Geometry: final body of the model. Coordinates: model frame, mm. A direction names the side the tool comes from. Coordinates: 2 decimals unless noted, no trailing zeros. Loops run counter-clockwise (first coordinate to the right, second up) from the corner with the lowest first, then second, coordinate; pieces in that order, holes last. Notation, with made-up numbers: (86.5, 5) - (107.5, 5) arc R14 cw to (107.5, 28) - close; hole circle Ø6 at (-12, 47). An arc over 180 degrees is marked (long way). Answer in a Markdown table with one row per item.
from build123d import *

# Parameters (mm, degrees)
ESQUISSE1_W             = 600
ESQUISSE1_H             = 480
BOSS_EXTRU_1_DEPTH      = 18
ESQUISSE2_W             = 100
ESQUISSE2_H             = 79
ENL_V_MAT_EXTRU_1_DEPTH = 17
ENL_V_MAT_EXTRU_3_DEPTH = 10
CONG_1_R                = 2


with BuildPart() as part:
    # Esquisse1 → Boss.-Extru.1 (new body)
    with BuildSketch(Plane.XY):
        Rectangle(ESQUISSE1_W, ESQUISSE1_H)
    extrude(amount=BOSS_EXTRU_1_DEPTH)

    # Esquisse2 → Enlèv. mat.-Extru.1 (cut)
    with BuildSketch(Plane.XY.offset(18)):
        with Locations((40, 9.5)):
            Rectangle(ESQUISSE2_W, ESQUISSE2_H)
    extrude(amount=-ENL_V_MAT_EXTRU_1_DEPTH, mode=Mode.SUBTRACT)

    # Esquisse4 → Enlèv. mat.-Extru.3 (cut)
    with BuildSketch(Plane.XY.offset(1)):
        Polygon((75, 49), (5, 49), (5, 34), (-10, 34), (-10, -15), (5, -15), (5, -30), (75, -30), (75, -15), (90, -15), (90, 34), (75, 34), align=None)
    extrude(amount=-ENL_V_MAT_EXTRU_3_DEPTH, mode=Mode.SUBTRACT)

    # Congé1
    cong_1_edges = [part.edges().sort_by_distance(p)[0] for p in [
        (5, -15, 0.5),
        (5, 34, 0.5),
        (75, 34, 0.5),
        (75, -15, 0.5),
    ]]
    fillet(cong_1_edges, radius=CONG_1_R)


solid = part.part
(1) First-contact query: pin 1 Ø7.5 at (x, y) = (-5, -25.5) entering from +Z. Flat tip, straight axial feed; report the tip coordinate or a pass-through.
Verdict:
| item | result |
|---|---|
| pin 1 | stops at z = 1 |
(2) Cut plane A-A on z = 4.5. Output: boundary loops of the cut face in (x, y).
Verdict:
| item | result |
|---|---|
| outline | (-300, -240) - (300, -240) - (300, 240) - (-300, 240) - close; hole (-10, -30) - (90, -30) - (90, 49) - (-10, 49) - close |
(3) Access query for faces 1 (the face through (-4, 57, 18)), 2 (the face through (82, 42, 1)). Directions: +Z, -Z, +X, -X, +Y, -Y. A direction counts if a zero-diameter tool reaches every point of the face in a straight line with its end or side. Return the directions, or none.
Verdict:
| item | result |
|---|---|
| face 1 | +Z, +X, -X, +Y, -Y |
| face 2 | +Z |
(4) Ray query, probe 1 along Y at (x, z) = (32.5, 6.25); probe 2 along X at (y, z) = (36.5, 3.75). Return the intervals inside material, ascending.
Verdict:
| item | result |
|---|---|
| probe 1 | y = -240 to -30, 49 to 240 |
| probe 2 | x = -300 to -10, 90 to 300 |
(5) Pull-direction query (Y, two-part tool) for faces 3 (the face through (-4, 240, 9)), 4 (the face through (-4, -240, 9)), 5 (the face through (-10, 10, 9)), 6 (the face through (-4, 57, 0)); classes: pulls with the +Y half, pulls with the -Y half, needs draft (parallel to the pull), parting line crosses it, or undercut.
Verdict:
| item | result |
|---|---|
| face 3 | pulls with the +Y half |
| face 4 | pulls with the -Y half |
| face 5 | undercut |
| face 6 | needs draft |
